Design review of the part built by this model. Coordinates are the model's own, in mm. A direction names the side the tool comes from. Coordinates: 2 decimals unless noted, no trailing zeros. Write each loop counter-clockwise with the first axis right and the second up, starting at its lowest first coordinate (ties: lowest second). Pieces come first, ordered by that corner, then holes. Notation, with made-up numbers: (20, -5) -> (45, -5) arc R22 ccw to (45, 4) -> close; hole circle Ø7 at (64.5, 22.5). An arc over 180 degrees is marked (long way). One line per question, with ' | ' between items. Start each with the question number.
Q1. For P1, Ø1.8, axis at x = 96, z = 25.5, coming from the -Y side; P2, Ø5, axis at y = 39, z = 25.5, coming from the -X side; P3, Ø6, axis at y = 70, z = 24.5, coming from the +X side, all flat-tipped, find the tip position at first contact; note any pin that passes through.
Q2. For faces 1 (the flat face through (84, 26, 25)), 2 (the flat face through (16, 50, 25)), 3 (the flat face through (84, 74, 25)), 4 (the flat face through (154, 50, 25)), 5 (the flat face through (84, 100, 10)), list the 3-axis set-ups (+Z, -Z, +X, -X, +Y, -Y) from which the entire face can be reached by the end or side of a thin tool; tool diameter is ignored.
Q3. Add section B-B on y = 80.5. State the section outline as (x, z) points.
Q4. Add section C-C on z = 24.25. State the section outline as (x, y) points.
Q5. Add section A-A on x = 128.5. State the section outline as (y, z) points, and give its area (3 significant figures).
Q6. Add section D-D on y = 41.5. State the section outline as (x, z) points.
Q7. Wall thickness on probe 1 along Z at (x, y) = (145, 86.5); probe 2 along Y at (x, z) = (34.5, 24.5); probe 3 along X at (y, z) = (87.5, 20.25): over which ranges is each line inside the solid? List them lowest first.
from build123d import *

# Parameters (mm, degrees)
SKETCH_W     = 170
SKETCH_H     = 100
PAD_DEPTH    = 21
SKETCH001_W  = 138
SKETCH001_H  = 48
PAD001_DEPTH = 8
FILLET_R     = 1
FILLET001_R  = 1
FILLET002_R  = 1


with BuildPart() as part:
    # Sketch → Pad (new body)
    with BuildSketch(Plane.XY):
        with Locations((85, 50)):
            Rectangle(SKETCH_W, SKETCH_H)
    extrude(amount=PAD_DEPTH)

    # Sketch001 (on Face6 of Pad) → Pad001 (join)
    with BuildSketch(Plane.XY.offset(21)):
        with Locations((85, 50)):
            Rectangle(SKETCH001_W, SKETCH001_H)
    extrude(amount=PAD001_DEPTH)

    # Fillet
    fillet_edges = [part.edges().sort_by_distance(p)[0] for p in [
        (85, 26, 29),
        (154, 50, 29),
        (85, 74, 29),
        (16, 50, 29),
    ]]
    fillet(fillet_edges, radius=FILLET_R)

    # Fillet001
    fillet001_edges = [part.edges().sort_by_distance(p)[0] for p in [
        (85, 0, 21),
        (0, 50, 21),
        (170, 50, 21),
        (85, 100, 21),
        (85, 26, 21),
        (154, 50, 21),
        (85, 74, 21),
        (16, 50, 21),
    ]]
    fillet(fillet001_edges, radius=FILLET001_R)

    # Fillet002
    fillet002_edges = [part.edges().sort_by_distance(p)[0] for p in [
        (85, 0, 0),
        (170, 50, 0),
        (85, 100, 0),
        (0, 50, 0),
    ]]
    fillet(fillet002_edges, radius=FILLET002_R)


solid = part.part
Output values:
1) P1: stops at y = 26 | P2: stops at x = 16 | P3: stops at x = 154.13
2) face 1: +Z, +X, -X, -Y | face 2: +Z, -X, +Y, -Y | face 3: +Z, +X, -X, +Y | face 4: +Z, +X, +Y, -Y | face 5: +Z, -Z, +X, -X, +Y
3) outline: (0, 1) arc R1 ccw to (1, 0) -> (169, 0) arc R1 ccw to (170, 1) -> (170, 20) arc R1 ccw to (169, 21) -> (1, 21) arc R1 ccw to (0, 20) -> close
4) outline: (16, 26) -> (154, 26) -> (154, 74) -> (16, 74) -> close
5) outline: (0, 1) arc R1 ccw to (1, 0) -> (99, 0) arc R1 ccw to (100, 1) -> (100, 20) arc R1 ccw to (99, 21) -> (75, 21) arc R1 cw to (74, 22) -> (74, 28) arc R1 ccw to (73, 29) -> (27, 29) arc R1 ccw to (26, 28) -> (26, 22) arc R1 cw to (25, 21) -> (1, 21) arc R1 ccw to (0, 20) -> close | area: 2,480 mm2
6) outline: (0, 1) arc R1 ccw to (1, 0) -> (169, 0) arc R1 ccw to (170, 1) -> (170, 20) arc R1 ccw to (169, 21) -> (155, 21) arc R1 cw to (154, 22) -> (154, 28) arc R1 ccw to (153, 29) -> (17, 29) arc R1 ccw to (16, 28) -> (16, 22) arc R1 cw to (15, 21) -> (1, 21) arc R1 ccw to (0, 20) -> close
7) probe 1: z = 0 to 21 | probe 2: y = 26 to 74 | probe 3: x = 0.03 to 169.97
